from build123d import *

# Parameters (mm, degrees)
SKETCH1_W                                       = 80
SKETCH1_H                                       = 80
EXTRUDE1_DEPTH                                  = 10
CBORE_FOR_10_SOCKET_HEAD_CAP_SCREW2_D           = 5.1054
CBORE_FOR_10_SOCKET_HEAD_CAP_SCREW2_CBORE_D     = 9.525
CBORE_FOR_10_SOCKET_HEAD_CAP_SCREW2_CBORE_DEPTH = 4.826
M3X0_5_TAPPED_HOLE1_AT_2_COUNT                  = 2
M3X0_5_TAPPED_HOLE1_AT_2_PITCH                  = 50.4
LPATTERN4_COUNT                                 = 2
LPATTERN4_PITCH                                 = 25.2


with BuildPart() as part:
    # Sketch1 → Extrude1 (new body)
    with BuildSketch(Plane.XY):
        with Locations((-15.736421911, 19.385081585)):
            Rectangle(SKETCH1_W, SKETCH1_H)
    extrude(amount=EXTRUDE1_DEPTH)

    # CBORE for #10 Socket Head Cap Screw2 (through all)
    with Locations(Plane(origin=(-47.486421911, 44.077855478, 10), x_dir=(1, 0, 0), z_dir=(0, 0, 1))):
        with Locations((0, 0), (0, -25.4), (0, -50.8), (63.5, -50.8), (63.5, -25.4), (63.5, 0)):
            CounterBoreHole(CBORE_FOR_10_SOCKET_HEAD_CAP_SCREW2_D / 2, CBORE_FOR_10_SOCKET_HEAD_CAP_SCREW2_CBORE_D / 2, CBORE_FOR_10_SOCKET_HEAD_CAP_SCREW2_CBORE_DEPTH)

    # Sketch4 → M3x0.5 Tapped Hole1 (revolve, cut)
    with BuildSketch(Plane(origin=(-28.336421911, 34.785081585, 10), x_dir=(0, -1, 0), z_dir=(1, 0, 0))):
        Polygon((0, 0), (0, 8.251075774), (1.25, 7.5), (1.25, 6), (1.5, 6), (1.5, 0), align=None)
    m3x0_5_tapped_hole1 = revolve(axis=Axis((-28.336421911, 34.785081585, 16.35), (0, 0, -1)), mode=Mode.SUBTRACT)

    # M3x0.5 Tapped Hole1 at 2: M3x0.5 Tapped Hole1 ×2
    with Locations(*[(0, -i * M3X0_5_TAPPED_HOLE1_AT_2_PITCH, 0) for i in range(1, M3X0_5_TAPPED_HOLE1_AT_2_COUNT)]):
        add(m3x0_5_tapped_hole1, mode=Mode.SUBTRACT)

    # LPattern4: M3x0.5 Tapped Hole1 ×2
    with Locations(*[(i * LPATTERN4_PITCH, 0, 0) for i in range(1, LPATTERN4_COUNT)]):
        add(m3x0_5_tapped_hole1, mode=Mode.SUBTRACT)

    # LPattern4 copy 1 sketch → LPattern4 copy 1 (revolve, cut)
    with BuildSketch(Plane(origin=(-3.136421911, -15.614918415, 10), x_dir=(0, -1, 0), z_dir=(1, 0, 0))):
        Polygon((0, 0), (0, 8.251075774), (1.25, 7.5), (1.25, 6), (1.5, 6), (1.5, 0), align=None)
    revolve(axis=Axis((-3.136421911, -15.614918415, 16.35), (0, 0, -1)), mode=Mode.SUBTRACT)


solid = part.part
The model under review builds one solid part; all positions refer to its coordinate system, in mm. A direction names the side the tool comes from. Round coordinates to 2 decimals unless told otherwise and drop trailing zeros. Write each loop counter-clockwise with the first axis right and the second up, starting at its lowest first coordinate (ties: lowest second). Pieces come first, ordered by that corner, then holes. Notation, with made-up numbers: M -23,70.5 L -3,70.5 A26 ccw -3,84.5 Z; hole C -18,-2 d11. An arc over 180 degrees is marked long. Answer as CSV lines item,"result". Start each with the question number.
Q1. Wall thickness on line 1 along X through (y, z) = (35, 8.25); line 2 along X through (y, z) = (-6.5, 7.25); line 3 along Y through (x, z) = (-48, 9.25): over which ranges is each line inside the solid? List them lowest first.
Q2. The part is to be moulded in two halves that separate along Y. For faces 3 (the face through (-16, 59.385, 5)), 4 (the face through (24.264, 19, 5)), 5 (the face through (-16, -20.615, 5)), 6 (the face through (-3.28, -15.45, 1.88)), say which applies: +Y half, -Y half, draft (parallel to the pull), parting line (faces both ways), or undercut.
Q3. Clearance check with flat-ended pins moving along their axes: P1, Ø2.5, axis at x = -28.5, y = -16, coming from the +Z side; P2, Ø5.5, axis at x = 16.01, y = -6.72, coming from the +Z side; P3, Ø2.5, axis at x = -3, y = -15.5, coming from the +Z side; P4, Ø4, axis at x = -47.49, y = -6.72, coming from the -Z side. State where each tip first meets the part, or that it passes through.
Q4. Tool access review of faces 1 (the face through (-16, 20, 0)), 2 (the face through (-3.202, 36.284, 7.042)): name each direction out of +Z, -Z, +X, -X, +Y, -Y from which nothing blocks a thin tool from reaching the whole face with its end or side.
Q5. Consider section A-A, the plane x = 17. Give the boundary of the cut face in (y, z), then the cut area to 3 significant figures.
Q6. Consider section B-B, the plane z = 6.75. State how many separate pieces and enclosed holes the cut face has, then the cut area to 3 significant figures.
Result set:
1,line 1,"x = -55.74 to -29.82, -26.85 to -4.62, -1.65 to 24.26"
1,line 2,"x = -55.74 to -52.24, -42.73 to 11.26, 20.77 to 24.26"
1,line 3,"y = -20.61 to -11.46, -1.99 to 13.94, 23.41 to 39.34, 48.81 to 59.39"
2,face 3,"+Y half"
2,face 4,"draft"
2,face 5,"-Y half"
2,face 6,"undercut"
3,P1,"stops at z = 10"
3,P2,"stops at z = 5.17"
3,P3,"stops at z = 4"
3,P4,"passes through"
4,face 1,"-Z, +X, -X, +Y, -Y"
4,face 2,"+Z"
5,outline,"M -20.61,0 L -9.08,0 L -9.08,5.17 L -11.38,5.17 L -11.38,10 L -20.61,10 Z; M -4.37,0 L 16.32,0 L 16.32,5.17 L 14.02,5.17 L 14.02,10 L -2.06,10 L -2.06,5.17 L -4.37,5.17 Z; M 21.03,0 L 41.72,0 L 41.72,5.17 L 39.42,5.17 L 39.42,10 L 23.34,10 L 23.34,5.17 L 21.03,5.17 Z; M 46.43,0 L 59.39,0 L 59.39,10 L 48.74,10 L 48.74,5.17 L 46.43,5.17 Z"
5,area,"592 mm²"
6,separate pieces,"1"
6,enclosed holes,"10"
6,area,"5,940 mm²"
